Build history of the part. All positions in model axes, mm. Face numbers are marked on the shaded views. Coordinates: 2 decimals unless noted, no trailing zeros. Loops run counter-clockwise (first coordinate to the right, second up) from the corner with the lowest first, then second, coordinate; pieces in that order, holes last.
(1) Slice it at C-C (z = 17). Give the cut face in (x, y) (1 decimal), and give its area (3 significant figures).
(2) Flat gauge pin, fed straight in: P1, Ø5, axis at y = 7.5, z = 12.5, coming from the -X side. Where does the tip first touch, or does it go through?
(3) Slice it at D-D (x = -37). Give the cut face in (y, z).
(4) Slice it at A-A (x = -13). Give the cut face in (y, z), and give its area (3 significant figures).
(5) Two-plate mould, pull along X, no slides. Class the marked faces 1, 2, 3 and 4: pulls with the +X half, pulls with the -X half, needs draft (parallel to the pull), parting line crosses it, or undercut.
(6) Wall check: L1, parallel to Y at x = -31, z = 32; L2, parallel to X at y = 9, z = 21.5; L3, parallel to Y at x = -1, z = 34.5. Give the ranges that are in metal, low to high.
(7) Slice it at B-B (y = 29). Give the cut face in (x, z).
from build123d import *

# Parameters (mm, degrees)
F0_R     = 9.20886
F1_DEPTH = 66.3
F2_R     = 5


with BuildPart() as f1:
    # F0 (on Top) → F1 (new body)
    with BuildSketch(Plane.XY):
        with BuildLine():
            Line((13.70497, 36.908648), (-44.589408, 36.908648))
            Line((-44.589408, 36.908648), (-44.589408, 20))
            ThreePointArc((-44.589408, 20), (-38.731543, 5.857864), (-24.589408, 0))
            Line((-24.589408, 0), (-6.29503, 0))
            ThreePointArc((-6.29503, 0), (7.847106, 5.857864), (13.70497, 20))
            Line((13.70497, 20), (13.70497, 36.908648))
        make_face()
        with Locations((-24.90058, 10.326985)):
            Circle(F0_R, mode=Mode.SUBTRACT)
        with Locations((-5.98386, 9.940929)):
            Circle(F0_R, mode=Mode.SUBTRACT)
        with Locations((-34.551967, 26.541315)):
            Circle(F0_R, mode=Mode.SUBTRACT)
        with Locations((-15.442219, 26.734345)):
            Circle(F0_R, mode=Mode.SUBTRACT)
        with Locations((3.474499, 26.348287)):
            Circle(F0_R, mode=Mode.SUBTRACT)
    extrude(amount=F1_DEPTH)

    # F2
    f2_edges = [f1.edges().sort_by_distance(p)[0] for p in [
        (13.70497, 36.908648, 33.15),
        (-44.589408, 36.908648, 33.15),
    ]]
    fillet(f2_edges, radius=F2_R)


solid = f1.part
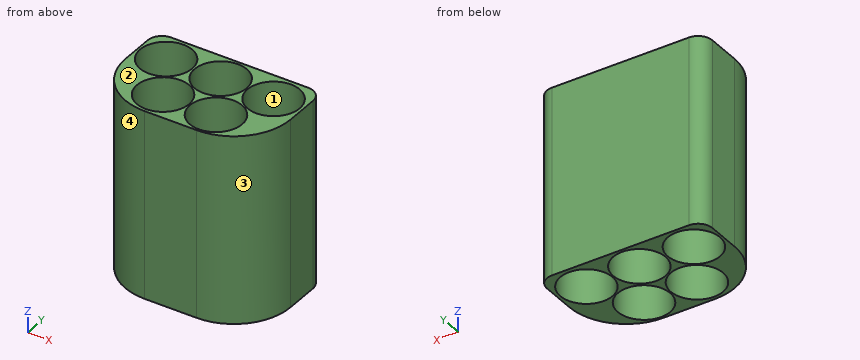
Response values:
1. outline: (-44.6, 20) arc R20 ccw to (-24.6, 0) - (-6.3, 0) arc R20 ccw to (13.7, 20) - (13.7, 31.9) arc R5 ccw to (8.7, 36.9) - (-39.6, 36.9) arc R5 ccw to (-44.6, 31.9) - close; hole circle Ø18.4 at (-34.6, 26.5); hole circle Ø18.4 at (-24.9, 10.3); hole circle Ø18.4 at (-15.4, 26.7); hole circle Ø18.4 at (-6, 9.9); hole circle Ø18.4 at (3.5, 26.3)
1. area: 637 mm2
2. P1: stops at x = -41.91
3. outline: (4.32, 0) - (17.66, 0) - (17.66, 66.3) - (4.32, 66.3) - close; (35.42, 0) - (36.91, 0) - (36.91, 66.3) - (35.42, 66.3) - close
4. outline: (0, 0) - (3.98, 0) - (3.98, 66.3) - (0, 66.3) - close; (15.91, 0) - (17.86, 0) - (17.86, 66.3) - (15.91, 66.3) - close; (35.61, 0) - (36.91, 0) - (36.91, 66.3) - (35.61, 66.3) - close
4. area: 479 mm2
5. face 1: undercut
5. face 2: needs draft
5. face 3: pulls with the +X half
5. face 4: pulls with the -X half
6. L1: y = 1.06 to 3.43, 17.23 to 18.05, 35.04 to 36.91
6. L2: x = -41.29 to -34.01, -15.79 to -15.14, 3.18 to 10.41
6. L3: y = 0.71 to 2.2, 17.68 to 18.3, 34.4 to 36.91
7. outline: (-44.59, 0) - (-43.43, 0) - (-43.43, 66.3) - (-44.59, 66.3) - close; (-25.68, 0) - (-24.37, 0) - (-24.37, 66.3) - (-25.68, 66.3) - close; (-6.52, 0) - (-5.34, 0) - (-5.34, 66.3) - (-6.52, 66.3) - close; (12.29, 0) - (13.7, 0) - (13.7, 66.3) - (12.29, 66.3) - close
